Autodesk Inventor part; units mm, degrees
ref_plane "YZ Plane" through (0, 0, 0) normal (1, 0, 0) x (0, 1, 0)
ref_plane "XZ Plane" through (0, 0, 0) normal (0, 1, 0) x (-1, 0, 0)
ref_plane "XY Plane" through (0, 0, 0) normal (0, 0, 1) x (1, 0, 0)
sketch "Skizze1" plane through (0, 0, 0) normal (0, 1, 0) x (-1, 0, 0)
  circle A0 centre (0, 0) radius 100
  circle A1 centre (0, 0) radius 95.1
  line L0 (100, 0) -> (-150, 0) construction
  line L1 (-91.6515, 40) -> (-150, 40)
  line L2 (-150, 40) -> (-150, -40)
  line L3 (-150, -40) -> (-91.6515, -40)
  dimension "d0" = 200
  dimension "d1" = 4.9
  dimension "d2" = 150
  dimension "d3" = 80
extrude "Extrusion1" add sketch "Skizze1" along normal mid plane 80 contours A0 L3 L2 L1
sketch "Skizze2" plane through (150, -40, -40) normal (1, 0, 0) x (0, 0, -1)
  circle A0 centre (-40, 40) radius 36.5
  line L0 (-72.5, 7.5) -> (-7.5, 7.5)
  line L1 (-7.5, 7.5) -> (-7.5, 72.5)
  line L2 (-7.5, 72.5) -> (-72.5, 72.5)
  line L3 (-72.5, 72.5) -> (-72.5, 7.5)
  line L4 (-72.5, 7.5) -> (-7.5, 72.5) construction
  line L5 (-7.5, 7.5) -> (-72.5, 72.5) construction
  circle A1 centre (-72.5, 72.5) radius 3
  circle A2 centre (-7.5, 72.5) radius 3
  circle A3 centre (-7.5, 7.5) radius 3
  circle A4 centre (-72.5, 7.5) radius 3
  point P0 (-40, 40)
  dimension "d6" = 73
  dimension "d9" = 65
  dimension "d10" = 6
extrude "Extrusion2" cut sketch "Skizze2" against normal through all contours A0 L1 | L1 A0 L0 L3 L2 | L2 A0 | A2 L2 L1 | L1 L2 A2 | A0 L0 | A3 L0 L1 | L1 L0 A3 | L3 A0 | A1 L3 L2 | L2 L3 A1 | A4 L3 L0 | L0 L3 A4
equation "\"d0\" = kg_diameter"
equation "\"d1\" = kg_thickness"
equation "\"d4\" = d3"
equation "\"d6\" = bore_diameter"
equation "\"kg_diameter\" = 200"
equation "\"kg_thickness\" = 4.9"
equation "\"ht_thickness\" = 1.9"
equation "\"case_thickness\" = 18"
equation "\"gap_fit\" = 0.1"
equation "\"gap_slide\" = 0.2"
equation "\"gap_air\" = 1"
equation "\"bore_diameter\" = 73"
properties part number "Bohrhilfe"
Can you work these out from the model? Positions are in its coordinate system, mm. Give positions to 0.01 mm unless a question says otherwise; leave off trailing zeros. Write each loop counter-clockwise with the first axis right and the second up, starting at its lowest first coordinate (ties: lowest second). Pieces come first, ordered by that corner, then holes. Notation, with made-up numbers: (33.5, 82.25) -> (73.5, 82.25) arc R4 ccw to (73.5, 88.25) -> close; hole circle Ø2 at (9, 59). An arc over 180 degrees is marked (long way). Write item = value, one per line.
(1) Suppose I cut it at B-B on y = -32.5. Write out the boundary of the cut face in (x, z).
Worked out:
outline = (91.65, -40) -> (150, -40) -> (150, -35.5) -> (93.49, -35.5) arc R100 cw to start; (91.65, 40) arc R100 cw to (93.49, 35.5) -> (150, 35.5) -> (150, 40) -> close; (95.55, -29.5) -> (150, -29.5) -> (150, -16.61) -> (98.61, -16.61) arc R100 cw to start; (95.55, 29.5) arc R100 cw to (98.61, 16.61) -> (150, 16.61) -> (150, 29.5) -> close
(2) I'm going to push a flat-ended pin straight in: P1, Ø7, axis at y = -32.5, z = -32.5, coming from the -X side. Where does the tip first touch, or does it pass through?
Worked out:
P1 = 93.3
(3) Suppose I cut it at A-A on z = 0. Write out the boundary of the cut face in (x, y).
Worked out:
outline = (100, -40) -> (150, -40) -> (150, -36.5) -> (100, -36.5) -> close; (100, 36.5) -> (150, 36.5) -> (150, 40) -> (100, 40) -> close
(4) I need wall thicknesses on probe 1 along Y at (x, z) = (116, 0); probe 2 along Y at (x, z) = (107, -33); probe 3 along Y at (x, z) = (103.5, 21.5). Which ranges of each line are inside material? Lowest first, please. Write a range as from..to.
Worked out:
probe_1 = -40..-36.5, 36.5..40
probe_2 = -40..-35.46, -29.54..-15.6, 15.6..29.54, 35.46..40
probe_3 = -40..-29.5, 29.5..40
(5) Thinking about a two-plate mould opening in Z: for faces 1 (the face through (121, -1, -40)), 2 (the face through (122.1, -32.4, 35.5)), 3 (the face through (150, 18, 33)), which applies, released by +Z, released by -Z, zero draft, split by the parting line, or undercut?
Worked out:
face_1 = released by -Z
face_2 = undercut
face_3 = zero draft
(6) Suppose I cut it at C-C on x = 123.5. Write out the boundary of the cut face in (y, z), then the cut area to 3 significant figures.
Worked out:
outline = (-40, -40) -> (40, -40) -> (40, 40) -> (-40, 40) -> close; hole circle Ø73 at (0, 0); hole circle Ø6 at (-32.5, -32.5); hole circle Ø6 at (-32.5, 32.5); hole circle Ø6 at (32.5, -32.5); hole circle Ø6 at (32.5, 32.5)
area = 2,100 mm^2
(7) Suppose I cut it at D-D on y = -14.5. Write out the boundary of the cut face in (x, z).
Worked out:
outline = (91.65, -40) -> (150, -40) -> (150, -33.5) -> (94.22, -33.5) arc R100 cw to start; (91.65, 40) arc R100 cw to (94.22, 33.5) -> (150, 33.5) -> (150, 40) -> close
